Could you check a few things on this model? Use its own coordinates, in mm. A direction names the side the tool comes from. Give positions to 0.01 mm unless a question says otherwise; leave off trailing zeros. Loops run counter-clockwise (first coordinate to the right, second up) from the corner with the lowest first, then second, coordinate; pieces in that order, holes last. Notation, with made-up numbers: M -28.5,27 L -5.5,27 A17 ccw -5.5,53 Z; hole C -2,87 d1. An arc over 180 degrees is marked long. Use a Markdown table: item, result. Add a question column.
1) We'd pull the mould along Z, two halves only. Please class faces 1 (the cylindrical face through (6.44, 49.12, 23.76)), 2 (the flat face through (8, -60, 38.1)), 3 (the flat face through (9, -63.5, -1)): +Z half, -Z half, draft (parallel to the pull), parting line (faces both ways), or undercut.
2) If I drill on line 1 along X through (y, z) = (13.5, -30); line 2 along Z through (x, y) = (-10, 0.5); line 3 along Y through (x, z) = (9.5, -20.5), over which ranges is the centre line in solid material (lowest first)? Write a range as [from, to].
3) Suppose I cut it at A-A on z = 0. List the corners of the cut face in (x, y) for me, and give its area (3 significant figures).
4) Suppose I cut it at C-C on z = -19.05. List the corners of the cut face in (x, y) for me.
5) Suppose I cut it at D-D on x = 3. List the corners of the cut face in (y, z) for me.
6) Suppose I cut it at B-B on y = 0. List the corners of the cut face in (x, z) for me.
7) Which directions (+Z, -Z, +X, -X, +Y, -Y) give clear straight access to the entire face, cutting with the end or side of a thin tool? Please do faces 4 (the flat face through (-33.02, 0, 0)), 5 (the cylindrical face through (-16.457, 2.304, 10.375)), 6 (the flat face through (0, -14, -7)).
8) Will these pins go through, and if not, where does the flat tip stop? pin 1 Ø16.5 at (y, z) = (-56.79, -19.05) entering from -X; pin 2 Ø3 at (x, z) = (-4.5, -1.5) entering from +Y; pin 3 Ø8 at (x, z) = (-1, -26) entering from -Y.
```python
from build123d import *

# Parameters (mm, degrees)
F0_W        = 127
F0_H        = 76.2
F1_DEPTH    = 12.7
F2_R        = 6.35
F3_DEPTH    = 12.701
F4_W        = 7.6199990327
F4_H        = 10.6278949787
F6_R        = 2.54
F7_C1_SIZE  = 5.08
F7_T2_DEPTH = 153.1282991577
F7_T4_DEPTH = 97.2482991577
F7_T6_DEPTH = 92.1682991577


# Not quite as in the source:
# - a fillet or chamfer that OpenCascade refuses, or shapes differently, is made with other operations: its cross-section is extruded or revolved along the edge and cut away or added
# - a feature names something its author has since deleted; it is built from what else it names


with BuildPart() as f1:
    # F0 (on Right) → F1 (new body)
    with BuildSketch(Plane.YZ):
        Rectangle(F0_W, F0_H)
    extrude(amount=F1_DEPTH)

    # F2 (on face) → F3 (cut, through all)
    with BuildSketch(Plane.YZ.offset(12.7)):
        with BuildLine():
            ThreePointArc((-56.6875480297, 38.1), (-58.333550533, 26.9256825374), (-48.2882989585, 32.089752231))
            ThreePointArc((-48.2882989585, 32.089752231), (-49.4742292648, 35.7850038056), (-52.5890498873, 38.1))
            Line((-52.5890498873, 38.1), (-56.6875480297, 38.1))
        make_face()
        with Locations((-56.7933163234, -19.05)):
            Circle(F2_R)
        with Locations((52.4994003593, -29.1107435445)):
            Circle(F2_R)
        with Locations((43.2542454979, 26.190802066)):
            Circle(F2_R)
    extrude(amount=-F3_DEPTH, mode=Mode.SUBTRACT)

    # F4 (on Top) → F5 (revolve)
    with BuildSketch(Plane.XY):
        Polygon((-20.3199990327, -10.6278949787), (-20.3199990327, 0), (-33.0199990327, 0), (-33.0199990327, -12.7), (-20.3199990327, -12.7), align=None)
        with Locations((-16.5099995164, -5.3139474893)):
            Rectangle(F4_W, F4_H)
        Polygon((0, 0), (-12.7, 0), (-12.7, -10.6278949787), (-12.7, -12.7), (0, -12.7), align=None)
    revolve(axis=Axis((-26.6699990327, 0, 0), (1, 0, 0)))

    # F6
    f6_edges = [f1.edges().sort_by_distance(p)[0] for p in [
        (-33.019999, 12.7, 0),
        (0, 12.7, 0),
    ]]
    fillet(f6_edges, radius=F6_R)

    # F7: chamfer of 5.08 on 4 edges, made by hand

    # F7_c1
    f7_c1_edges = [f1.edges().sort_by_distance(p)[0] for p in [
        (0, 5.4554750563, 38.1),
    ]]
    chamfer(f7_c1_edges, length=F7_C1_SIZE)

    # F7_s3 → F7_t2 (cut)
    with BuildSketch(Plane.XZ.offset(-76.5641495789)):
        with BuildLine():
            Line((-0.1436840979, -32.8763159021), (5.2236840979, -38.2436840979))
            Line((5.2236840979, -38.2436840979), (5.2236840979, -38.3452840979))
            ThreePointArc((5.2236840979, -38.3452840979), (2.611842049, -38.2016), (0, -38.2016))
            Line((0, -38.2016), (-0.1016, -38.1))
            ThreePointArc((-0.1016, -38.1), (-0.1016, -35.488157951), (-0.2452840979, -32.8763159021))
            Line((-0.2452840979, -32.8763159021), (-0.1436840979, -32.8763159021))
        make_face()
    extrude(amount=F7_T2_DEPTH, mode=Mode.SUBTRACT)

    # F7_s5 → F7_t4 (cut)
    with BuildSketch(Plane.XY.offset(-46.0841495789)):
        with BuildLine():
            Line((-0.1436840979, -58.2763159021), (5.2236840979, -63.6436840979))
            Line((5.2236840979, -63.6436840979), (5.2236840979, -63.7452840979))
            ThreePointArc((5.2236840979, -63.7452840979), (2.611842049, -63.6016), (0, -63.6016))
            Line((0, -63.6016), (-0.1016, -63.5))
            ThreePointArc((-0.1016, -63.5), (-0.1016, -60.888157951), (-0.2452840979, -58.2763159021))
            Line((-0.2452840979, -58.2763159021), (-0.1436840979, -58.2763159021))
        make_face()
    extrude(amount=F7_T4_DEPTH, mode=Mode.SUBTRACT)

    # F7_s7 → F7_t6 (cut)
    with BuildSketch(Plane.XY.offset(-46.0841495789)):
        with BuildLine():
            Line((-0.1436840979, 58.2763159021), (5.2236840979, 63.6436840979))
            Line((5.2236840979, 63.6436840979), (5.2236840979, 63.7452840979))
            ThreePointArc((5.2236840979, 63.7452840979), (2.611842049, 63.6016), (0, 63.6016))
            Line((0, 63.6016), (-0.1016, 63.5))
            ThreePointArc((-0.1016, 63.5), (-0.1016, 60.888157951), (-0.2452840979, 58.2763159021))
            Line((-0.2452840979, 58.2763159021), (-0.1436840979, 58.2763159021))
        make_face()
    extrude(amount=F7_T6_DEPTH, mode=Mode.SUBTRACT)


solid = f1.part
```
Answer block:
| question | item | result |
|---|---|---|
| 1 | face 1 | undercut |
| 1 | face 2 | +Z half |
| 1 | face 3 | draft |
| 2 | line 1 | x = [0, 12.7] |
| 2 | line 2 | z = [-12.69, 12.69] |
| 2 | line 3 | y = [-63.5, -62.98], [-50.61, 63.5] |
| 3 | outline | M -33.02,-10.16 A2.54 ccw -30.48,-12.7 L -20.32,-12.7 L -20.32,-10.63 L -12.7,-10.63 L -12.7,-12.7 L -2.54,-12.7 A2.54 cw 0,-15.24 L 0,-58.42 L 5.08,-63.5 L 12.7,-63.5 L 12.7,63.5 L 5.08,63.5 L 0,58.42 L 0,15.24 A2.54 cw -2.54,12.7 L -12.7,12.7 L -12.7,10.63 L -20.32,10.63 L -20.32,12.7 L -30.48,12.7 A2.54 ccw -33.02,10.16 Z |
| 3 | area | 2,390 mm^2 |
| 4 | outline | M 0,-50.44 L 12.7,-50.44 L 12.7,63.5 L 5.08,63.5 L 0,58.42 Z; M 4.72,-63.14 L 5.08,-63.5 L 12.7,-63.5 L 12.7,-63.14 Z |
| 5 | outline | M -61.42,-36.02 L 61.42,-36.02 L 61.42,36.02 L -49.65,36.02 A6.35 cw long -56.69,38.1 L -61.42,38.1 L -61.42,-14.7 A6.35 cw long -61.42,-23.4 Z; hole C 43.25,26.19 d12.7; hole C 52.5,-29.11 d12.7 |
| 6 | outline | M -33.02,-10.16 A2.54 ccw -30.48,-12.7 L -20.32,-12.7 L -20.32,-10.63 L -12.7,-10.63 L -12.7,-12.7 L -2.54,-12.7 A2.54 cw 0,-15.24 L 0,-33.02 L 5.08,-38.1 L 12.7,-38.1 L 12.7,38.1 L 5.08,38.1 L 0,33.02 L 0,15.24 A2.54 cw -2.54,12.7 L -12.7,12.7 L -12.7,10.63 L -20.32,10.63 L -20.32,12.7 L -30.48,12.7 A2.54 ccw -33.02,10.16 Z |
| 7 | face 4 | +Z, -Z, -X, +Y, -Y |
| 7 | face 5 | none |
| 7 | face 6 | -X |
| 8 | pin 1 | stops at x = 0 |
| 8 | pin 2 | stops at y = 12.7 |
| 8 | pin 3 | stops at y = -61.42 |
